Read the model definition and answer for the solid it produces. Units are mm, in the model's axes. A direction names the side the tool comes from. Round coordinates to 2 decimals unless told otherwise and drop trailing zeros. Loops run counter-clockwise (first coordinate to the right, second up) from the corner with the lowest first, then second, coordinate; pieces in that order, holes last. Notation, with made-up numbers: M 54.25,61.5 L 65.25,61.5 A17 ccw 65.25,90.5 Z; hole C 58.25,-16 d10. An arc over 180 degrees is marked long. Write each question's results on one line, items separated by ' | '.
from build123d import *

# Parameters (mm, degrees)
BOSS_EXTRUDE1_DEPTH = 20
SKETCH2_R           = 26.722222222
SKETCH2_R_2         = 17.722222222
BOSS_EXTRUDE2_DEPTH = 20
CUT_EXTRUDE1_DEPTH  = 65
SKETCH4_R           = 15
BOSS_EXTRUDE3_DEPTH = 65
CIRPATTERN1_COUNT   = 4


with BuildPart() as part:
    # Sketch1 → Boss-Extrude1 (new body, symmetric)
    with BuildSketch(Plane.XY):
        with BuildLine():
            ThreePointArc((0, -25), (-25, 0), (0, 25))
            Line((0, 25), (9, 25))
            Line((9, 25), (9, 45))
            Line((9, 45), (0, 45))
            ThreePointArc((0, 45), (-23.717082451, 38.242646352), (-40.311288741, 20))
            Line((-40.311288741, 20), (-140.311288741, 20))
            Line((-140.311288741, 20), (-140.311288741, -20))
            Line((-140.311288741, -20), (-40.311288741, -20))
            ThreePointArc((-40.311288741, -20), (-23.717082451, -38.242646352), (0, -45))
            Line((0, -45), (9, -45))
            Line((9, -45), (9, -25))
            Line((9, -25), (0, -25))
        make_face()
    extrude(amount=BOSS_EXTRUDE1_DEPTH, both=True)

    # Sketch2 → Boss-Extrude2 (add)
    with BuildSketch(Plane(origin=(0, 45, 0), x_dir=(1, 0, 0), z_dir=(0, 1, 0))):
        with Locations((26.722222222, 0)):
            Circle(SKETCH2_R)
        with Locations((26.722222222, 0)):
            Circle(SKETCH2_R_2, mode=Mode.SUBTRACT)
    boss_extrude2 = extrude(amount=-BOSS_EXTRUDE2_DEPTH)

    # Mirror1: Boss-Extrude2 across plane
    add(boss_extrude2.mirror(Plane.ZX))

    # Sketch3 → Cut-Extrude1 (cut)
    with BuildSketch(Plane.ZY.offset(140.311288741)):
        Polygon((-12.5, 20), (-20, 20), (-20, 12.5), align=None)
    cut_extrude1 = extrude(amount=-CUT_EXTRUDE1_DEPTH, mode=Mode.SUBTRACT)

    # Sketch4 → Boss-Extrude3 (add)
    with BuildSketch(Plane.ZY.offset(140.311288741)):
        Circle(SKETCH4_R)
    extrude(amount=BOSS_EXTRUDE3_DEPTH)

    # CirPattern1: Cut-Extrude1 ×4 about axis
    cirpattern1_axis = Axis((0, 0, 0), (1, 0, 0))
    for i in range(1, CIRPATTERN1_COUNT):
        add(cut_extrude1.rotate(cirpattern1_axis, i * 360 / CIRPATTERN1_COUNT), mode=Mode.SUBTRACT)


solid = part.part
Item 1: The part is cut by section C-C (x = -118.5). Determine the outline of the cut face in (y, z), plus the area to 3 significant figures.
Outcome:
outline: M -20,-12.5 L -12.5,-20 L 12.5,-20 L 20,-12.5 L 20,12.5 L 12.5,20 L -12.5,20 L -20,12.5 Z | area: 1,490 mm2
Item 2: The part is cut by section A-A (z = 0). Determine the outline of the cut face in (x, y).
Outcome:
outline: M -205.31,-15 L -140.31,-15 L -140.31,-20 L -40.31,-20 A45 ccw 0,-45 L 9,-45 L 9,-25 L 0,-25 A25 cw 0,25 L 9,25 L 9,45 L 0,45 A45 ccw -40.31,20 L -140.31,20 L -140.31,15 L -205.31,15 Z; M 44.44,-45 L 53.44,-45 L 53.44,-25 L 44.44,-25 Z; M 44.44,25 L 53.44,25 L 53.44,45 L 44.44,45 Z
Item 3: Straight lines are drawn through the part: line 1 (Z direction, x = -42, y = -18); line 2 (Y direction, x = 9, z = 11.5); line 3 (X direction, y = -31.5, z = -12). For each, find the intervals that lie inside material, in ascending order.
Outcome:
line 1: z = -20 to 20 | line 2: y = -45 to -25, 25 to 45 | line 3: x = -32.14 to 13.68, 39.76 to 50.6
Item 4: The mould has two halves that part along Z. Classify faces 1 (the face through (12.658, 35.14, 10.784)), 2 (the face through (-75.311, 17, 17)), 3 (the face through (-50, 1, 20)), 4 (the face through (-108.3, 16.2, -16.3)): pulls with the +Z half, pulls with the -Z half, needs draft (parallel to the pull), parting line crosses it, or undercut.
Outcome:
face 1: undercut | face 2: needs draft | face 3: pulls with the +Z half | face 4: pulls with the -Z half
Item 5: For faces 5 (the face through (-79, 20, 0)), 6 (the face through (-75.311, -17, 17)), 7 (the face through (-140.311, -9, 14)), 8 (the face through (-75.311, -17, -17)), 9 (the face through (8.5, 25, -0.4)), determine the directions among +Z, -Z, +X, -X, +Y, -Y from which every point of the face is accessible in a straight line to the end or side of a thin tool.
Outcome:
face 5: +Z, -Z, -X, +Y | face 6: +Z, -X, -Y | face 7: -X | face 8: -Z, -X, -Y | face 9: +Z, -Z, +X
Item 6: The part is cut by section B-B (y = 0). Determine the outline of the cut face in (x, z), plus the area to 3 significant figures.
Outcome:
outline: M -205.31,-15 L -140.31,-15 L -140.31,-20 L -25,-20 L -25,20 L -140.31,20 L -140.31,15 L -205.31,15 Z | area: 6,560 mm2
Item 7: Flat-ended cylindrical pins translate along their axes: pin 1 (8.5 mm diameter, centred on y = 15, z = 17, fed in from -X); pin 2 (4 mm diameter, centred on x = -153.5, z = 1, fed in from +Y); pin 3 (6 mm diameter, centred on x = -26.5, y = -4, fed in from +Z); pin 4 (10 mm diameter, centred on x = -16.5, y = -2, fed in from +Z). Find the tip coordinate at first contact, or state that the pin passes through.
Outcome:
pin 1: stops at x = -140.31 | pin 2: stops at y = 15 | pin 3: stops at z = 20 | pin 4: passes through
Item 8: The part is cut by section D-D (y = 36). Determine the outline of the cut face in (x, z).
Outcome:
outline: M -27,-20 L 9,-20 A26.72 ccw long 9,20 L -27,20 Z; hole C 26.72,0 d35.44
